from build123d import *

# Parameters (mm, degrees)
EXTRUDE_1_DEPTH          = 112
SKETCH_3_W               = 140
SKETCH_3_H               = 140
EXTRUDE_2_DEPTH          = 2
EXTRUDE_3_DEPTH          = 1
CUT_EXTRUDE_1_DEPTH      = 2
PATTERN_CIRCULAR_2_COUNT = 4
SKETCH_7_R               = 5
CUT_EXTRUDE_2_DEPTH      = 150.479095528
SKETCH_8_W               = 10.222107434
SKETCH_8_H               = 48.162502517
CUT_EXTRUDE_3_DEPTH      = 112


with BuildPart() as part:
    # 草图1 → 凸台-拉伸1 (new body)
    with BuildSketch(Plane(origin=(0, 0, 0), x_dir=(1, 0, 0), z_dir=(0, 1, 0))):
        with BuildLine():
            Line((-19.5, -22.5), (19.5, -22.5))
            ThreePointArc((19.5, -22.5), (21.621320344, -21.621320344), (22.5, -19.5))
            Line((22.5, -19.5), (22.5, 19.5))
            ThreePointArc((22.5, 19.5), (21.621320344, 21.621320344), (19.5, 22.5))
            Line((19.5, 22.5), (-19.5, 22.5))
            ThreePointArc((-19.5, 22.5), (-21.621320344, 21.621320344), (-22.5, 19.5))
            Line((-22.5, 19.5), (-22.5, -19.5))
            ThreePointArc((-22.5, -19.5), (-21.621320344, -21.621320344), (-19.5, -22.5))
        make_face()
        with BuildLine():
            Line((-19.5, -20.5), (19.5, -20.5))
            ThreePointArc((19.5, -20.5), (20.207106781, -20.207106781), (20.5, -19.5))
            Line((20.5, -19.5), (20.5, 19.5))
            ThreePointArc((20.5, 19.5), (20.207106781, 20.207106781), (19.5, 20.5))
            Line((19.5, 20.5), (-19.5, 20.5))
            ThreePointArc((-19.5, 20.5), (-20.207106781, 20.207106781), (-20.5, 19.5))
            Line((-20.5, 19.5), (-20.5, -19.5))
            ThreePointArc((-20.5, -19.5), (-20.207106781, -20.207106781), (-19.5, -20.5))
        make_face(mode=Mode.SUBTRACT)
    extrude(amount=EXTRUDE_1_DEPTH)

    # 草图3 → 凸台-拉伸2 (add)
    with BuildSketch(Plane.XZ):
        Rectangle(SKETCH_3_W, SKETCH_3_H)
    extrude(amount=EXTRUDE_2_DEPTH)

    # 草图4 → 凸台-拉伸3 (add, symmetric)
    with BuildSketch(Plane.XY):
        Polygon((22.5, 32), (42.5, 0), (22.5, 0), align=None)
    extrude(amount=EXTRUDE_3_DEPTH, both=True)

    # 草图6 → 切除-拉伸1 (cut)
    with BuildSketch(Plane.XY.offset(22.5)):
        with BuildLine():
            Line((-4.1, 80), (-4.1, 92))
            ThreePointArc((-4.1, 92), (0, 96.1), (4.1, 92))
            Line((4.1, 92), (4.1, 80))
            ThreePointArc((4.1, 80), (0, 75.9), (-4.1, 80))
        make_face()
        with BuildLine():
            Line((-4.1, 20), (-4.1, 32))
            ThreePointArc((-4.1, 32), (0, 36.1), (4.1, 32))
            Line((4.1, 32), (4.1, 20))
            ThreePointArc((4.1, 20), (0, 15.9), (-4.1, 20))
        make_face()
    cut_extrude_1 = extrude(amount=-CUT_EXTRUDE_1_DEPTH, mode=Mode.SUBTRACT)

    # 阵列(圆周)2: 切除-拉伸1 ×4 about axis, 1 skipped
    pattern_circular_2_axis = Axis((0, 0, 0), (0, 1, 0))
    add([cut_extrude_1.rotate(pattern_circular_2_axis, i * 360 / PATTERN_CIRCULAR_2_COUNT) for i in range(1, PATTERN_CIRCULAR_2_COUNT) if i not in (1,)], mode=Mode.SUBTRACT)

    # 草图7 → 切除-拉伸2 (cut, through all)
    with BuildSketch(Plane(origin=(0, 0, 0), x_dir=(1, 0, 0), z_dir=(0, 1, 0))):
        with Locations(Location((50, 50, 0), (0, 0, 270))):
            Circle(SKETCH_7_R)
        with Locations(Location((50, -50, 0), (0, 0, 270))):
            Circle(SKETCH_7_R)
        with Locations(Location((-50, -50, 0), (0, 0, 270))):
            Circle(SKETCH_7_R)
        with Locations(Location((-50, 50, 0), (0, 0, 270))):
            Circle(SKETCH_7_R)
    extrude(amount=-CUT_EXTRUDE_2_DEPTH, mode=Mode.SUBTRACT)

    # 草图8 → 切除-拉伸3 (cut)
    with BuildSketch(Plane(origin=(0, 112, 0), x_dir=(1, 0, 0), z_dir=(0, 1, 0))):
        with Locations((-24.611053717, 1.581251259)):
            Rectangle(SKETCH_8_W, SKETCH_8_H)
    extrude(amount=-CUT_EXTRUDE_3_DEPTH, mode=Mode.SUBTRACT)


solid = part.part
Model file for the job. Use its own axes, mm. A direction names the side the tool comes from. Coordinates: 2 decimals unless noted, no trailing zeros. Write each loop counter-clockwise with the first axis right and the second up, starting at its lowest first coordinate (ties: lowest second). Pieces come first, ordered by that corner, then holes. Notation, with made-up numbers: (23, 83) - (82, 83) arc R16 ccw to (82, 87) - close; hole circle Ø10 at (76.5, 49). An arc over 180 degrees is marked (long way). Write each question's results on one line, items separated by ' | '. Start each with the question number.
1) Cut at A-A (x = 0). Write the cut outline in (y, z), then the cut area to 3 significant figures.
2) Cut at B-B (z = -50). Write the cut outline in (x, y), then the cut area to 3 significant figures.
3) 3-axis set-ups, long thin cutter, end or side, ignore diameter. For faces 4 (the face through (0, 55, -22.5)), 5 (the face through (0.1, 36.1, -21.5)), 6 (the face through (0, 55, -20.5)), 7 (the face through (28, 9, 1)): which of +Z, -Z, +X, -X, +Y, -Y reach the whole face in a straight line?
4) Probe line 1 along X through (y, z) = (-1, 50); line 2 along Z through (x, y) = (15.5, 81); line 3 along Y through (x, z) = (61.5, 5.5). List the from-to ranges inside material, lowest first. Write a range as from..to.
5) Mould opens along Y. For faces 1 (the face through (-1, 0, 1)), 2 (the face through (0, 55, 20.5)), 3 (the face through (0.1, 96.1, -21.5)) say: pulls with the +Y half, pulls with the -Y half, needs draft (parallel to the pull), parting line crosses it, or undercut.
6) Flat gauge pins, fed straight in: P1, Ø11.5, axis at y = 28.5, z = 2, coming from the -X side; P2, Ø4, axis at y = 45.5, z = -25, coming from the -X side; P3, Ø2, axis at y = 86.5, z = 21, coming from the +X side; P4, Ø19.5, axis at x = 3.5, y = 73.5, coming from the +Z side. Where does each tip first touch, or does it go through?
7) Cut at D-D (y = 85). Write the cut outline in (x, z), then the cut area to 3 significant figures.
8) Cut at C-C (x = -50). Write the cut outline in (y, z), then the cut area to 3 significant figures.
Returned:
1) outline: (-2, -70) - (0, -70) - (0, -22.5) - (15.9, -22.5) - (15.9, -20.5) - (0, -20.5) - (0, 20.5) - (15.9, 20.5) - (15.9, 22.5) - (0, 22.5) - (0, 70) - (-2, 70) - close; (36.1, -22.5) - (75.9, -22.5) - (75.9, -20.5) - (36.1, -20.5) - close; (36.1, 20.5) - (75.9, 20.5) - (75.9, 22.5) - (36.1, 22.5) - close; (96.1, -22.5) - (112, -22.5) - (112, -20.5) - (96.1, -20.5) - close; (96.1, 20.5) - (112, 20.5) - (112, 22.5) - (96.1, 22.5) - close | area: 566 mm^2
2) outline: (-70, -2) - (-55, -2) - (-55, 0) - (-70, 0) - close; (-45, -2) - (45, -2) - (45, 0) - (-45, 0) - close; (55, -2) - (70, -2) - (70, 0) - (55, 0) - close | area: 240 mm^2
3) face 4: -Z, +X, -X, +Y | face 5: +Z, -Z | face 6: -X, +Y | face 7: +Z, +X, +Y
4) line 1: -70..-55, -45..45, 55..70 | line 2: -22.5..-20.5, 20.5..22.5 | line 3: -2..0
5) face 1: pulls with the +Y half | face 2: needs draft | face 3: undercut
6) P1: x = 20.5 | P2: through | P3: x = 22.46 | P4: z = 22.5
7) outline: (-19.5, -22.5) - (-4.1, -22.5) - (-4.1, -20.5) - (-19.5, -20.5) - close; (-19.5, 20.5) - (-4.1, 20.5) - (-4.1, 22.5) - (-19.5, 22.5) - close; (4.1, -22.5) - (19.5, -22.5) arc R3 ccw to (22.5, -19.5) - (22.5, 19.5) arc R3 ccw to (19.5, 22.5) - (4.1, 22.5) - (4.1, 20.5) - (19.5, 20.5) arc R1 cw to (20.5, 19.5) - (20.5, -19.5) arc R1 cw to (19.5, -20.5) - (4.1, -20.5) - close | area: 214 mm^2
8) outline: (-2, -70) - (0, -70) - (0, -55) - (-2, -55) - close; (-2, -45) - (0, -45) - (0, 45) - (-2, 45) - close; (-2, 55) - (0, 55) - (0, 70) - (-2, 70) - close | area: 240 mm^2
